Part model, mm, in its own coordinate system. A direction names the side the tool comes from. Give positions to 0.01 mm unless a question says otherwise; leave off trailing zeros. Order: outer loops, then holes, each group sorted by start corner. A loop starts at its lowest first (then second) coordinate and runs counter-clockwise, first axis right, second up. Notation, with made-up numbers: (-38.75, -33.75) - (-6.75, -33.75) arc R24 ccw to (-6.75, -21.75) - close; hole circle Ø1 at (80, 36). An arc over 180 degrees is marked (long way). Use one line per item in the form item = value. Start each with the question number.
1. Pin check, flat tips, straight feed: P1, Ø1.7, axis at x = 7, y = 0, coming from the -Z side; P2, Ø1.2, axis at x = 0, z = -1, coming from the -Y side; P3, Ø2, axis at y = -3, z = 0.5, coming from the -X side. Stop position of each tip, or through.
2. Tool access for faces 1 (the face through (0, 8.524, -1)), 2 (the face through (0, -8.524, -1)), 3 (the face through (6.15, 6.25, -0.74)): list every direction of +Z, -Z, +X, -X, +Y, -Y with a clear straight run to the whole face (end or side of a thin tool).
3. Pull direction Y, two halves, no side cores. Call faces 4 (the face through (-0.54, -2.44, 3.88)), 5 (the face through (-11, 1.875, -1)), 6 (the face through (0, -2, 2.3)), 7 (the face through (-10, 0, -37.5)): +Y half, -Y half, draft (parallel to the pull), parting line (faces both ways), or undercut.
4. Band-saw the part on A-A, the plane y = -7. List the corners of the cut face in (x, z).
5. Band-saw the part on B-B, the plane x = 0. List the corners of the cut face in (y, z), plus the area to 3 significant figures.
6. Drill centre lines: line 1 (Z direction, x = -2, y = 3.25); line 2 (Z direction, x = -3.5, y = -6.5); line 3 (X direction, y = 7, z = 0.05). Where is each one in solid material? Low to high.
7. Band-saw the part on D-D, the plane x = -11. List the corners of the cut face in (y, z) (3 decimals).
from build123d import *

# Parameters (mm, degrees)
SKETCH1_R           = 10.5
BOSS_EXTRUDE1_DEPTH = 2.3
SKETCH2_R           = 0.75
CUT_EXTRUDE1_DEPTH  = 16.026310259
SKETCH3_R           = 1.5
CUT_EXTRUDE2_DEPTH  = 2.3
CIRPATTERN1_COUNT   = 4
SKETCH4_R           = 4.4
SKETCH4_R_2         = 2.5
BOSS_EXTRUDE2_DEPTH = 3.2
SKETCH5_W           = 22
SKETCH5_H           = 3.75
SKETCH5_R           = 0.75
SKETCH5_R_2         = 1.5
BOSS_EXTRUDE3_DEPTH = 1.5
SKETCH6_R           = 1.778
BOSS_EXTRUDE4_DEPTH = 36
SKETCH7_W           = 3.75
SKETCH7_H           = 6.6491
SKETCH7_R           = 0.75
BOSS_EXTRUDE5_DEPTH = 1.5


with BuildPart() as part:
    # Sketch1 → Boss-Extrude1 (new body)
    with BuildSketch(Plane.XY):
        Circle(SKETCH1_R)
    extrude(amount=BOSS_EXTRUDE1_DEPTH)

    # Sketch2 → Cut-Extrude1 (cut, through all)
    with BuildSketch(Plane.XY.offset(2.3)):
        with Locations((0, 7)):
            Circle(SKETCH2_R)
    cut_extrude1 = extrude(amount=-CUT_EXTRUDE1_DEPTH, mode=Mode.SUBTRACT)

    # Sketch3 → Cut-Extrude2 (cut)
    with BuildSketch(Plane.XY.offset(2.3)):
        Circle(SKETCH3_R)
    extrude(amount=-CUT_EXTRUDE2_DEPTH, mode=Mode.SUBTRACT)

    # CirPattern1: Cut-Extrude1 ×4 about axis
    cirpattern1_axis = Axis((0, 0, 0), (0, 0, 1))
    for i in range(1, CIRPATTERN1_COUNT):
        add(cut_extrude1.rotate(cirpattern1_axis, i * 360 / CIRPATTERN1_COUNT), mode=Mode.SUBTRACT)

    # Sketch4 → Boss-Extrude2 (add)
    with BuildSketch(Plane.XY.offset(2.3)):
        Circle(SKETCH4_R)
        Circle(SKETCH4_R_2, mode=Mode.SUBTRACT)
    extrude(amount=BOSS_EXTRUDE2_DEPTH)

    # Sketch5 → Boss-Extrude3 (add)
    with BuildSketch(Plane(origin=(0, 0, 0), x_dir=(-1, 0, 0), z_dir=(0, 0, -1))):
        with Locations((2.475846117, 0)):
            Rectangle(SKETCH5_W, SKETCH5_H)
        with Locations(Location((7, 0, 0), (0, 0, 90))):
            Circle(SKETCH5_R, mode=Mode.SUBTRACT)
        with Locations(Location((-7, 0, 0), (0, 0, 270))):
            Circle(SKETCH5_R, mode=Mode.SUBTRACT)
        with Locations(Location((0, 0, 0), (0, 0, 180))):
            Circle(SKETCH5_R_2, mode=Mode.SUBTRACT)
    extrude(amount=BOSS_EXTRUDE3_DEPTH)

    # Sketch6 → Boss-Extrude4 (add)
    with BuildSketch(Plane(origin=(0, 0, -1.5), x_dir=(-1, 0, 0), z_dir=(0, 0, -1))):
        with Locations((10.16, 0)):
            Circle(SKETCH6_R)
    extrude(amount=BOSS_EXTRUDE4_DEPTH)

    # Sketch7 → Boss-Extrude5 (add)
    with BuildSketch(Plane(origin=(0, 0, 0), x_dir=(-1, 0, 0), z_dir=(0, 0, -1))):
        with BuildLine():
            Line((-8.524153883, 1.875), (-1.875, 1.875))
            Line((-1.875, 1.875), (-1.875, 8.5241))
            ThreePointArc((-1.875, 8.5241), (-6.199356528, 6.199337688), (-8.524153883, 1.875))
        make_face()
        with BuildLine():
            Line((1.875, 8.5241), (1.875, 1.875))
            Line((1.875, 1.875), (8.5241, 1.875))
            ThreePointArc((8.5241, 1.875), (6.199324729, 6.199324729), (1.875, 8.5241))
        make_face()
        with BuildLine():
            Line((-1.875, -8.5241), (-1.875, -1.875))
            Line((-1.875, -1.875), (-8.524153883, -1.875))
            ThreePointArc((-8.524153883, -1.875), (-6.199356528, -6.199337688), (-1.875, -8.5241))
        make_face()
        with BuildLine():
            Line((8.5241, -1.875), (1.875, -1.875))
            Line((1.875, -1.875), (1.875, -8.5241))
            ThreePointArc((1.875, -8.5241), (6.199324729, -6.199324729), (8.5241, -1.875))
        make_face()
        with Locations((0, -5.19955)):
            Rectangle(SKETCH7_W, SKETCH7_H)
        with Locations((0, -7)):
            Circle(SKETCH7_R, mode=Mode.SUBTRACT)
        with Locations((0, 5.19955)):
            Rectangle(SKETCH7_W, SKETCH7_H)
        with Locations(Location((0, 7, 0), (0, 0, 180))):
            Circle(SKETCH7_R, mode=Mode.SUBTRACT)
    extrude(amount=BOSS_EXTRUDE5_DEPTH)


solid = part.part
From the geometry:
q1.P1 = -1.5
q1.P2 = -8.52
q1.P3 = -10.31
q2.face_1 = -Z, +X, -X, +Y
q2.face_2 = -Z, +X, -X, -Y
q2.face_3 = -Z, +X, +Y
q3.face_4 = undercut
q3.face_5 = +Y half
q3.face_6 = undercut
q3.face_7 = draft
q4.outline = (-7.83, 0) - (-5.27, 0) - (-5.27, -1.5) - (-0.75, -1.5) - (-0.75, 2.3) - (-7.83, 2.3) - close; (0.75, -1.5) - (5.27, -1.5) - (5.27, 0) - (7.83, 0) - (7.83, 2.3) - (0.75, 2.3) - close
q5.outline = (-10.5, 0) - (-8.52, 0) - (-8.52, -1.5) - (-7.75, -1.5) - (-7.75, 2.3) - (-10.5, 2.3) - close; (-6.25, -1.5) - (-1.5, -1.5) - (-1.5, 2.3) - (-2.5, 2.3) - (-2.5, 5.5) - (-4.4, 5.5) - (-4.4, 2.3) - (-6.25, 2.3) - close; (1.5, -1.5) - (6.25, -1.5) - (6.25, 2.3) - (4.4, 2.3) - (4.4, 5.5) - (2.5, 5.5) - (2.5, 2.3) - (1.5, 2.3) - close; (7.75, -1.5) - (8.52, -1.5) - (8.52, 0) - (10.5, 0) - (10.5, 2.3) - (7.75, 2.3) - close
q5.area = 63.2 mm²
q6.line_1 = -1.5 to 5.5
q6.line_2 = -1.5 to 2.3
q6.line_3 = -7.83 to -0.75, 0.75 to 7.83
q7.outline = (-1.875, -1.5) - (-1.567, -1.5) - (-1.567, -37.5) - (1.567, -37.5) - (1.567, -1.5) - (1.875, -1.5) - (1.875, 0) - (-1.875, 0) - close
